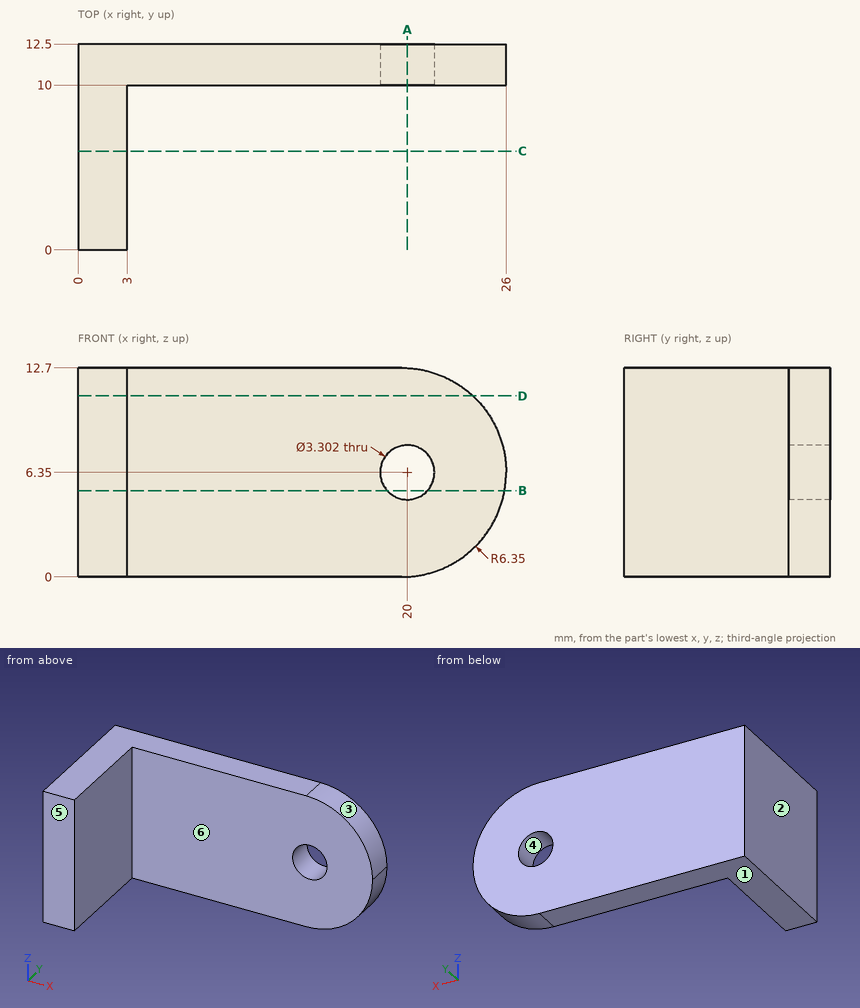
Answer from the drawing. Dimensions are ordinates in mm from the lowest x, y and z of the part. A direction names the side the tool comes from. Round coordinates to 2 decimals unless told otherwise and drop trailing zeros. Write each loop counter-clockwise with the first axis right and the second up, starting at its lowest first coordinate (ties: lowest second). Pieces come first, ordered by that corner, then holes. Notation, with made-up numbers: (60, 75) - (91, 75) arc R9 ccw to (91, 82) - close; hole circle Ø8 at (25, 26). An arc over 180 degrees is marked (long way). Use a Markdown table: item, result.
(1) Each of these flat-tipped pins is pushed along its axis until it touches: pin 1 Ø2 at (y, z) = (7, 10.5) entering from +X; pin 2 Ø5 at (x, z) = (7, 2) entering from -Y. Where does it stop, or does it pass through?
Reported:
| item | result |
|---|---|
| pin 1 | x = 3 |
| pin 2 | y = 10 |
(2) Which of the six approach directions +Z, -Z, +X, -X, +Y, -Y give full straight-line access (tool end or side, diameter ignored) to the marked faces 5 and 6?
Reported:
| item | result |
|---|---|
| face 5 | +Z, -Z, +X, -X, -Y |
| face 6 | +Z, -Z, +X, -Y |
(3) The part is cut by section A-A (x = 20). Write down the section's boundary in (y, z), then the cut area to 3 significant figures.
Reported:
| item | result |
|---|---|
| outline | (10, 0.01) - (12.5, 0.01) - (12.5, 4.7) - (10, 4.7) - close; (10, 8) - (12.5, 8) - (12.5, 12.69) - (10, 12.69) - close |
| area | 23.4 mm2 |
(4) The part is cut by section B-B (z = 5.25). Write down the section's boundary in (x, y).
Reported:
| item | result |
|---|---|
| outline | (0, 0) - (3, 0) - (3, 10) - (18.77, 10) - (18.77, 12.5) - (0, 12.5) - close; (21.23, 10) - (25.9, 10) - (25.9, 12.5) - (21.23, 12.5) - close |
(5) Straight lines are drawn through the part: line 1 along Y through (x, z) = (22, 8); line 2 along X through (y, z) = (3.25, 1.75); line 3 along Z through (x, y) = (20, 11.15). For each, find the intervals that lie inside material, in ascending order. Write a range as [from, to].
Reported:
| item | result |
|---|---|
| line 1 | [10, 12.5] |
| line 2 | [0, 3] |
| line 3 | [0.01, 4.7], [8, 12.69] |
(6) The mould has two halves that part along Z. Classify the marked faces 1, 2, 3 and 4: released by +Z, released by -Z, zero draft, split by the parting line, or undercut.
Reported:
| item | result |
|---|---|
| face 1 | released by -Z |
| face 2 | zero draft |
| face 3 | released by +Z |
| face 4 | undercut |
(7) The part is cut by section C-C (y = 6). Write down the section's boundary in (x, z).
Reported:
| item | result |
|---|---|
| outline | (0, 0) - (3, 0) - (3, 12.7) - (0, 12.7) - close |
(8) The part is cut by section D-D (z = 11). Write down the section's boundary in (x, y).
Reported:
| item | result |
|---|---|
| outline | (0, 0) - (3, 0) - (3, 10) - (23.97, 10) - (23.97, 12.5) - (0, 12.5) - close |
